Verification items for the finished model (mm, model axes). A direction names the side the tool comes from. Round coordinates to 2 decimals unless told otherwise and drop trailing zeros. Order: outer loops, then holes, each group sorted by start corner. A loop starts at its lowest first (then second) coordinate and runs counter-clockwise, first axis right, second up. Notation, with made-up numbers: (46.5, 18.25) -> (85.5, 18.25) arc R29 cw to (85.5, 46.25) -> close; hole circle Ø2 at (-13, 56.5). An arc over 180 degrees is marked (long way). Return JSON: item names as keys, results as strings. Group by question number.
1) Tool access check on faces 1 (the flat face through (-3, 39.698, 19)), 2 (the cylindrical face through (-15.103, 17.054, 68.302)), 3 (the flat face through (-19, 29, 10)). Record the directions out of +Z, -Z, +X, -X, +Y, -Y that give a thin tool (end or side, any length) a straight path to the whole face; none if there is none.
2) Scan lines: L1, parallel to Z at x = -10, y = 25; L2, parallel to Z at x = -24.5, y = 34.5; L3, parallel to X at y = 40, z = 17. Record each from-to range of solid material in increasing order.
3) Section check A-A on y = 3.5. Enter the section's corners in (x, z), plus the area to 3 significant figures.
4) Section check B-B on z = 13. Enter the section's corners in (x, y), plus the area to 3 significant figures.
5) Depth check by flat-ended pin: pin 1 (8.5 mm diameter, centred on x = -14.5, z = 54, fed in from -Y); pin 2 (6.5 mm diameter, centred on x = -19.82, z = 50, fed in from +Y); pin 3 (2 mm diameter, centred on x = -16.5, z = 88, fed in from -Y); pin 4 (1 mm diameter, centred on y = -3.5, z = 81.5, fed in from +X). Enter the tip coordinate at first touch or a pass-through.
6) Section check C-C on x = -28. Enter the section's corners in (y, z), plus the area to 3 significant figures.
7) Draft check along Z on faces 4 (the flat face through (-31.84, 38.076, 16.046)), 5 (the flat face through (-15, 16.198, 85)), 6 (the flat face through (-35, 38, 21.26)), 7 (the cylindrical face through (-40, -29, 14)). Enter one of: pulls with the +Z half, pulls with the -Z half, needs draft (parallel to the pull), parting line crosses it, or undercut.
8) Section check D-D on y = -15. Enter the section's corners in (x, z).
```python
from build123d import *

# Parameters (mm, degrees)
F1_DEPTH     = 100
F2_W         = 15.6
F2_H         = 15.6
F3_DEPTH     = 134.9
F5_DEPTH     = 3.2
F6_R         = 2.025
F7_DEPTH     = 10
F8_R         = 3
F8_R_2       = 24.0417525773
F9_DEPTH     = 15
F10_R        = 49.99999
F11_W        = 18
F11_H        = 34.8
F12_DEPTH    = 100
F13_R        = 3.5
F14_DEPTH    = 50
F15_R        = 2.1
F16_DEPTH    = 25
F17_T1_DEPTH = 47.5
F17_T3_DEPTH = 47.5


# Not quite as in the source:
# - a fillet or chamfer that OpenCascade refuses, or shapes differently, is made with other operations: its cross-section is extruded or revolved along the edge and cut away or added
# - a fillet or chamfer is up to 0.001 mm smaller than in the source, because OpenCascade refuses the exact size


with BuildPart() as f1:
    # F0 (on Top) → F1 (new body)
    with BuildSketch(Plane.XY):
        Polygon((5.1774463622, 16.1983228068), (5.1774463622, 41.1983228068), (-44.8225536378, 41.1983228068), (-44.8225536378, -44.3016771932), (-34.8225536378, -44.3016771932), (-34.8225536378, 16.1983228068), align=None)
    extrude(amount=F1_DEPTH)

    # F2 (on face) → F3 (cut)
    with BuildSketch(Plane.YZ.offset(5.1774463622)):
        with Locations((28.6983228068, 17.8)):
            Rectangle(F2_W, F2_H)
        with Locations((28.6983228068, 82.2)):
            Rectangle(F2_W, F2_H)
    extrude(amount=-F3_DEPTH, mode=Mode.SUBTRACT)

    # F4 (on face) → F5 (cut)
    with BuildSketch(Plane.XZ.offset(-36.4983228068)):
        Polygon((-2.8249217064, 85.66), (-6.8201855692, 85.66), (-8.8178175006, 82.2), (-6.8201855692, 78.74), (-2.8249217064, 78.74), (-0.827289775, 82.2), align=None)
        Polygon((-32.8249217064, 85.66), (-36.8201855692, 85.66), (-38.8178175006, 82.2), (-36.8201855692, 78.74), (-32.8249217064, 78.74), (-30.827289775, 82.2), align=None)
        Polygon((-32.8249217064, 21.26), (-36.8201855692, 21.26), (-38.8178175006, 17.8), (-36.8201855692, 14.34), (-32.8249217064, 14.34), (-30.827289775, 17.8), align=None)
        Polygon((-2.8249217064, 21.26), (-6.8201855692, 21.26), (-8.8178175006, 17.8), (-6.8201855692, 14.34), (-2.8249217064, 14.34), (-0.827289775, 17.8), align=None)
    extrude(amount=-F5_DEPTH, mode=Mode.SUBTRACT)

    # F6 (on face) → F7 (cut)
    with BuildSketch(Plane(origin=(0, 41.1983228068, 0), x_dir=(-1, 0, 0), z_dir=(0, 1, 0))):
        with Locations((34.8225536378, 82.2)):
            Circle(F6_R)
        with Locations((4.8225536378, 17.8)):
            Circle(F6_R)
        with Locations((34.8225536378, 17.8)):
            Circle(F6_R)
        with Locations((4.8225536378, 82.2)):
            Circle(F6_R)
    extrude(amount=-F7_DEPTH, mode=Mode.SUBTRACT)

    # F8 (on face) → F9 (cut)
    with BuildSketch(Plane.YZ.offset(-34.8225536378)):
        with Locations((3.1983228068, 87)):
            Circle(F8_R)
        with Locations((3.1983228068, 13)):
            Circle(F8_R)
        with Locations((-35.6016771932, 50)):
            Circle(F8_R)
        with Locations((1.4400753841, 50)):
            Circle(F8_R_2)
    extrude(amount=-F9_DEPTH, mode=Mode.SUBTRACT)

    # F10 (radius 50 in the source; OpenCascade refuses exactly that, so slightly less here)
    f10_edges = [f1.edges().sort_by_distance(p)[0] for p in [
        (-39.822554, -44.301677, 100),
        (-39.822554, -44.301677, 0),
    ]]
    fillet(f10_edges, radius=F10_R)

    # F11 (on face) → F12 (cut)
    with BuildSketch(Plane.YZ.offset(-34.8225536378)):
        with Locations((25.1983228068, 50)):
            Rectangle(F11_W, F11_H)
    extrude(amount=F12_DEPTH, mode=Mode.SUBTRACT)

    # F13 (on face) → F14 (cut)
    with BuildSketch(Plane(origin=(0, 41.1983228068, 0), x_dir=(-1, 0, 0), z_dir=(0, 1, 0))):
        with Locations((19.8225536378, 0)):
            Circle(F13_R)
        with Locations((19.8225536378, 100)):
            Circle(F13_R)
    extrude(amount=-F14_DEPTH, mode=Mode.SUBTRACT)

    # F15 (on face) → F16 (cut)
    with BuildSketch(Plane(origin=(0, 41.1983228068, 0), x_dir=(-1, 0, 0), z_dir=(0, 1, 0))):
        with Locations((19.8225536378, 50)):
            Circle(F15_R)
        with Locations((19.8225536378, 60)):
            Circle(F15_R)
        with Locations((19.8225536378, 40)):
            Circle(F15_R)
        with Locations((4.8225536378, 50)):
            Circle(F15_R)
        with Locations((4.8225536378, 60)):
            Circle(F15_R)
        with Locations((4.8225536378, 40)):
            Circle(F15_R)
    extrude(amount=-F16_DEPTH, mode=Mode.SUBTRACT)

    # F17: fillet of radius 3 on 4 edges, made by hand

    # F17_s2 → F17_t1 (join)
    with BuildSketch(Plane.YZ.offset(-42.3225536378)):
        with BuildLine():
            ThreePointArc((31.1983228068, 67.4), (33.3196431503, 66.5213203436), (34.1983228068, 64.4))
            Line((34.1983228068, 64.4), (34.1983228068, 67.4))
            Line((34.1983228068, 67.4), (31.1983228068, 67.4))
        make_face()
        with BuildLine():
            ThreePointArc((31.1983228068, 32.6), (33.3196431503, 33.4786796564), (34.1983228068, 35.6))
            Line((34.1983228068, 35.6), (34.1983228068, 32.6))
            Line((34.1983228068, 32.6), (31.1983228068, 32.6))
        make_face()
    extrude(amount=F17_T1_DEPTH)

    # F17_s4 → F17_t3 (cut)
    with BuildSketch(Plane.YZ.offset(-34.8225536378)):
        with BuildLine():
            ThreePointArc((16.1983228068, 70.4), (17.0770024632, 68.2786796564), (19.1983228068, 67.4))
            Line((19.1983228068, 67.4), (16.1983228068, 67.4))
            Line((16.1983228068, 67.4), (16.1983228068, 70.4))
        make_face()
        with BuildLine():
            ThreePointArc((16.1983228068, 29.6), (17.0770024632, 31.7213203436), (19.1983228068, 32.6))
            Line((19.1983228068, 32.6), (16.1983228068, 32.6))
            Line((16.1983228068, 32.6), (16.1983228068, 29.6))
        make_face()
    extrude(amount=F17_T3_DEPTH, mode=Mode.SUBTRACT)


solid = f1.part
```
Check result:
{
 "1": {"face 1": "none", "face 2": "+X, -Y", "face 3": "+X, -X"},
 "2": {"L1": "0 to 10, 25.6 to 32.6, 67.4 to 74.4, 90 to 100", "L2": "0 to 10, 25.6 to 74.4, 90 to 100", "L3": "-44.82 to -36.68, -32.96 to -6.68, -2.96 to 5.18"},
 "3": {"outline": "(-44.82, 0.05) -> (-34.82, 0.05) -> (-34.82, 10.02) -> (-44.82, 10.02) -> close; (-44.82, 15.98) -> (-34.82, 15.98) -> (-34.82, 26.05) -> (-44.82, 26.05) -> close; (-44.82, 73.95) -> (-34.82, 73.95) -> (-34.82, 84.02) -> (-44.82, 84.02) -> close; (-44.82, 89.98) -> (-34.82, 89.98) -> (-34.82, 99.95) -> (-44.82, 99.95) -> close", "area": "401 mm^2"},
 "4": {"outline": "(-44.82, -27.93) -> (-34.82, -27.93) -> (-34.82, 0.2) -> (-44.82, 0.2) -> close; (-44.82, 6.2) -> (-34.82, 6.2) -> (-34.82, 16.2) -> (5.18, 16.2) -> (5.18, 20.9) -> (-44.82, 20.9) -> close; (-44.82, 36.5) -> (5.18, 36.5) -> (5.18, 41.2) -> (-44.82, 41.2) -> close", "area": "851 mm^2"},
 "5": {"pin 1": "y = 34.2", "pin 2": "y = 41.2", "pin 3": "y = 16.2", "pin 4": "x = -34.82"},
 "6": {"outline": "(16.2, 0) -> (41.2, 0) -> (41.2, 100) -> (16.2, 100) -> (16.2, 70.4) arc R3 ccw to (19.2, 67.4) -> (31.2, 67.4) arc R3 cw to (34.2, 64.4) -> (34.2, 35.6) arc R3 cw to (31.2, 32.6) -> (19.2, 32.6) arc R3 ccw to (16.2, 29.6) -> close; hole (20.9, 10) -> (36.5, 10) -> (36.5, 25.6) -> (20.9, 25.6) -> close; hole (20.9, 74.4) -> (36.5, 74.4) -> (36.5, 90) -> (20.9, 90) -> close", "area": "1,390 mm^2"},
 "7": {"face 4": "undercut", "face 5": "needs draft", "face 6": "undercut", "face 7": "pulls with the -Z half"},
 "8": {"outline": "(-44.82, 4.49) -> (-34.82, 4.49) -> (-34.82, 32.46) -> (-44.82, 32.46) -> close; (-44.82, 67.54) -> (-34.82, 67.54) -> (-34.82, 95.51) -> (-44.82, 95.51) -> close"}
}
